```python
from build123d import *

# Parameters (mm, degrees)
F1_DEPTH = 10
F2_D     = 5.25
F3_D     = 8
F4_R     = 5


with BuildPart() as f1:
    # F0 (on Top) → F1 (new body)
    with BuildSketch(Plane.XY):
        Polygon((0, 33.75), (0, 50.25), (-28, 50.25), (-28, -50.25), (-11.05, -50.25), (-11.05, -30.25), (0, -30.25), (0, -10.75), (-13.5, -10.75), (-13.5, 33.75), align=None)
        Polygon((11.05, -50.25), (28, -50.25), (28, 50.25), (0, 50.25), (0, 33.75), (13.5, 33.75), (13.5, -10.75), (0, -10.75), (0, -30.25), (11.05, -30.25), align=None)
        Polygon((-28, -50.25), (-28, 50.25), (-31, -30.25), (-31, -50.25), align=None)
        Polygon((28, 50.25), (28, -50.25), (31, -50.25), (31, -30.25), align=None)
    extrude(amount=F1_DEPTH)

    # F2 (through all)
    with Locations(Plane(origin=(0, 0, 0), x_dir=(1, 0, 0), z_dir=(0, 0, -1))):
        with Locations((20.6375, 20.25), (-20.6375, 20.25), (-20.6375, -33.75), (20.6375, -33.75), (-20.6375, -43.25), (20.6375, -43.25), (20.6375, 10.75), (-20.6375, 10.75)):
            Hole(F2_D / 2)

    # F3 (through all)
    with Locations(Plane(origin=(0, 0, 0), x_dir=(1, 0, 0), z_dir=(0, 0, -1))):
        with Locations((-19, 40.25), (19, 40.25)):
            Hole(F3_D / 2)

    # F4
    f4_edges = [f1.edges().sort_by_distance(p)[0] for p in [
        (28, 50.25, 5),
        (-28, 50.25, 5),
    ]]
    fillet(f4_edges, radius=F4_R)


solid = f1.part
```
Geometry check sheet. Reference: the model listing, model coordinates, mm. A direction names the side the tool comes from. Give positions to 0.01 mm unless a question says otherwise; leave off trailing zeros. Write each loop counter-clockwise with the first axis right and the second up, starting at its lowest first coordinate (ties: lowest second). Pieces come first, ordered by that corner, then holes.
1) Section check D-D, the plane x = 19. Record the boundary of the cut face in (y, z).
2) Gauge pin test, flat ends, axial feed: pin 1 (5 mm diameter, centred on y = 4.5, z = 2.5, fed in from -X); pin 2 (2 mm diameter, centred on y = 21.5, z = 1.5, fed in from +X); pin 3 (1.5 mm diameter, centred on y = 30.5, z = 2, fed in from +X). Record the tip position at first contact, or that the pin passes through.
3) Material ranges on L1, parallel to Y at x = 9.5, z = 7.75; L2, parallel to X at y = -18, z = 7; L3, parallel to X at y = -20.25, z = 6.5, recorded low to high.
4) Section check C-C, the plane z = 2. State how many separate pieces and enclosed holes the cut face has, and give its area (3 significant figures).
5) Access from +Z, -Z, +X, -X, +Y, -Y to the whole of each face (thin tool, end or side, straight path). Record for faces 5 (the flat face through (11.05, -40, 5)), 6 (the cylindrical face through (-18.479, -44.216, 5.07)).
6) Release check for a two-part mould opening along Y. For faces 1 (the flat face through (-13.5, 11, 5)), 2 (the flat face through (-29.57, 8.12, 4.93)), 3 (the flat face through (13.5, 12, 5)), 4 (the flat face through (-14, 1, 10)) record: pulls with the +Y half, pulls with the -Y half, needs draft (parallel to the pull), parting line crosses it, or undercut.
7) Section check B-B, the plane y = -35. Record the boundary of the cut face in (x, z), and give its area (3 significant figures).
8) Section check A-A, the plane x = -12. Record the boundary of the cut face in (y, z), and give its area (3 significant figures).
Computed:
1. outline: (-50.25, 0) - (-44.25, 0) - (-44.25, 10) - (-50.25, 10) - close; (-36.25, 0) - (-22.3, 0) - (-22.3, 10) - (-36.25, 10) - close; (-18.2, 0) - (-12.8, 0) - (-12.8, 10) - (-18.2, 10) - close; (-8.7, 0) - (31.7, 0) - (31.7, 10) - (-8.7, 10) - close; (35.8, 0) - (41.2, 0) - (41.2, 10) - (35.8, 10) - close; (45.3, 0) - (50.25, 0) - (50.25, 10) - (45.3, 10) - close
2. pin 1: stops at x = -29.8
2. pin 2: stops at x = 29.11
2. pin 3: stops at x = 28.76
3. L1: y = -30.25 to -10.75, 33.75 to 50.25
3. L2: x = -30.54 to -21.99, -19.29 to 19.29, 21.99 to 30.54
3. L3: x = -30.63 to -23.26, -18.01 to 18.01, 23.26 to 30.63
4. separate pieces: 1
4. enclosed holes: 11
4. area: 4,060 mm2
5. face 5: +Z, -Z, -Y
5. face 6: +Z, -Z
6. face 1: undercut
6. face 2: pulls with the +Y half
6. face 3: undercut
6. face 4: needs draft
7. outline: (-31, 0) - (-11.05, 0) - (-11.05, 10) - (-31, 10) - close; (11.05, 0) - (31, 0) - (31, 10) - (11.05, 10) - close
7. area: 399 mm2
8. outline: (-50.25, 0) - (-10.75, 0) - (-10.75, 10) - (-50.25, 10) - close; (33.75, 0) - (50.25, 0) - (50.25, 10) - (33.75, 10) - close
8. area: 560 mm2
